Here's how the part is built. I have some questions about the finished solid (model axes, mm). Coordinates: 2 decimals unless noted, no trailing zeros.
Item 1: Please list where these lines run through material, in increasing order: line 1 (X direction, y = 184.5, z = 8.5); line 2 (Z direction, x = -70, y = -102.5); line 3 (Z direction, x = 10.5, y = -122).
Item 2: I want a section at A-A (y = -1). Count the separate pieces of the cut face and the enclosed holes in it, and give its area (3 significant figures).
Item 3: I'm going to push flat-ended pins straight in: P1, Ø4.5, axis at x = -50, y = 26, coming from the +Z side; P2, Ø1.7, axis at y = -102.5, z = 0, coming from the -X side; P3, Ø6, axis at x = -31, z = 6.5, coming from the -Y side; P4, Ø0.5, axis at x = 19, y = 86, coming from the +Z side. Where does each tip first touch, or does it pass through?
from build123d import *

# Parameters (mm, degrees)
SKETCH_R  = 2.1
PAD_DEPTH = 250
FILLET_R  = 1.5


with BuildPart() as part:
    # Sketch → Pad (new body, symmetric)
    with BuildSketch(Plane.XZ):
        Polygon((-10, 10), (-3.1, 10), (-3.1, 8.2), (-6, 8.2), (-6, 7.06066), (-2.83934, 3.9), (2.83934, 3.9), (6, 7.06066), (6, 8.2), (3.1, 8.2), (3.1, 10), (16.9, 10), (16.9, 8.2), (14, 8.2), (14, 7.06066), (17.16066, 3.9), (22.83934, 3.9), (26, 7.06066), (26, 8.2), (23.1, 8.2), (23.1, 10), (36.9, 10), (36.9, 8.2), (34, 8.2), (34, 7.06066), (37.16066, 3.9), (42.83934, 3.9), (46, 7.06066), (46, 8.2), (43.1, 8.2), (43.1, 10), (56.9, 10), (56.9, 8.2), (54, 8.2), (54, 7.06066), (57.16066, 3.9), (62.83934, 3.9), (66, 7.06066), (66, 8.2), (63.1, 8.2), (63.1, 10), (76.9, 10), (76.9, 8.2), (74, 8.2), (74, 7.06066), (77.16066, 3.9), (82.83934, 3.9), (86, 7.06066), (86, 8.2), (83.1, 8.2), (83.1, 10), (90, 10), (90, 3.1), (88.2, 3.1), (88.2, 6), (87.06066, 6), (83.9, 2.83934), (83.9, -2.83934), (87.06066, -6), (88.2, -6), (88.2, -3.1), (90, -3.1), (90, -10), (83.1, -10), (83.1, -8.2), (86, -8.2), (86, -7.06066), (82.83934, -3.9), (77.16066, -3.9), (74, -7.06066), (74, -8.2), (76.9, -8.2), (76.9, -10), (63.1, -10), (63.1, -8.2), (66, -8.2), (66, -7.06066), (62.83934, -3.9), (57.16066, -3.9), (54, -7.06066), (54, -8.2), (56.9, -8.2), (56.9, -10), (43.1, -10), (43.1, -8.2), (46, -8.2), (46, -7.06066), (42.83934, -3.9), (37.16066, -3.9), (34, -7.06066), (34, -8.2), (36.9, -8.2), (36.9, -10), (23.1, -10), (23.1, -8.2), (26, -8.2), (26, -7.06066), (22.83934, -3.9), (17.16066, -3.9), (14, -7.06066), (14, -8.2), (16.9, -8.2), (16.9, -10), (3.1, -10), (3.1, -8.2), (6, -8.2), (6, -7.06066), (2.83934, -3.9), (-2.83934, -3.9), (-6, -7.06066), (-6, -8.2), (-3.1, -8.2), (-3.1, -10), (-10, -10), (-10, -3.1), (-8.2, -3.1), (-8.2, -6), (-7.06066, -6), (-3.9, -2.83934), (-3.9, 2.83934), (-7.06066, 6), (-8.2, 6), (-8.2, 3.1), (-10, 3.1), align=None)
        Circle(SKETCH_R, mode=Mode.SUBTRACT)
        with Locations((20, 0)):
            Circle(SKETCH_R, mode=Mode.SUBTRACT)
        with Locations((40, 0)):
            Circle(SKETCH_R, mode=Mode.SUBTRACT)
        with Locations((79.9, 0)):
            Circle(SKETCH_R, mode=Mode.SUBTRACT)
        with Locations((60, 0)):
            Circle(SKETCH_R, mode=Mode.SUBTRACT)
        Polygon((7.8, -6.53934), (4.1, -2.83934), (4.1, 2.83934), (7.8, 6.53934), (7.8, 8.2), (12.2, 8.2), (12.2, 6.53934), (15.9, 2.83934), (15.9, -2.83934), (12.2, -6.53934), (12.2, -8.2), (7.8, -8.2), align=None, mode=Mode.SUBTRACT)
        Polygon((27.8, 8.2), (27.8, 6.53934), (24.1, 2.83934), (24.1, -2.83934), (27.8, -6.53934), (27.8, -8.2), (32.2, -8.2), (32.2, -6.53934), (35.9, -2.83934), (35.9, 2.83934), (32.2, 6.53934), (32.2, 8.2), align=None, mode=Mode.SUBTRACT)
        Polygon((47.8, 8.2), (47.8, 6.53934), (44.1, 2.83934), (44.1, -2.83934), (47.8, -6.53934), (47.8, -8.2), (52.2, -8.2), (52.2, -6.53934), (55.9, -2.83934), (55.9, 2.83934), (52.2, 6.53934), (52.2, 8.2), align=None, mode=Mode.SUBTRACT)
        Polygon((72.2, -8.2), (72.2, -6.53934), (75.9, -2.83934), (75.9, 2.83934), (72.2, 6.53934), (72.2, 8.2), (67.8, 8.2), (67.8, 6.53934), (64.1, 2.83934), (64.1, -2.83934), (67.8, -6.53934), (67.8, -8.2), align=None, mode=Mode.SUBTRACT)
    extrude(amount=PAD_DEPTH, both=True)

    # Fillet
    fillet_edges = [part.edges().sort_by_distance(p)[0] for p in [
        (-10, 0, 10),
        (90, 0, 10),
        (90, 0, -10),
        (-10, 0, -10),
    ]]
    fillet(fillet_edges, radius=FILLET_R)


with BuildPart() as part_1:
    # Body placement: moved
    add(part.part.moved(Location((-70, 0, 0))))


solid = part_1.part
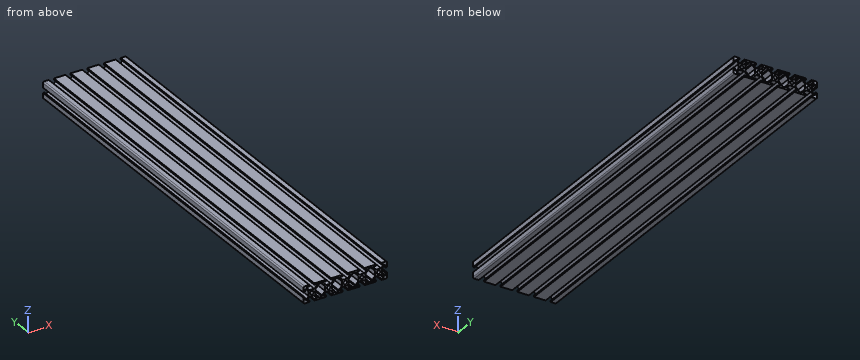
Answer:
1. line 1: x = -80 to -73.1, -66.9 to -53.1, -46.9 to -33.1, -26.9 to -13.1, -6.9 to 6.9, 13.1 to 20
1. line 2: z = -3.9 to -2.1, 2.1 to 3.9
1. line 3: z = -3.9 to -2.01, 2.01 to 3.9
2. separate pieces: 1
2. enclosed holes: 9
2. area: 729 mm2
3. P1: stops at z = 3.9
3. P2: stops at x = -73.9
3. P3: stops at y = -250
3. P4: stops at z = 9.98
